Verification items for the finished model (mm, model axes). A direction names the side the tool comes from. Give positions to 0.01 mm unless a question says otherwise; leave off trailing zeros. Loops run counter-clockwise (first coordinate to the right, second up) from the corner with the lowest first, then second, coordinate; pieces in that order, holes last. Notation, with made-up numbers: (43, 40) -> (82, 40) arc R6 cw to (82, 47) -> close; hole circle Ø5 at (19.25, -8). An arc over 180 degrees is marked (long way). Answer in a Markdown table with one row per item. Add a question column.
Q1. Section check A-A on z = 0. Enter the section's corners in (x, y).
Q2. Material ranges on probe 1 along Y at (x, z) = (-9, 0); probe 2 along Y at (x, z) = (9.5, -15.5); probe 3 along X at (y, z) = (4.75, -3), recorded low to high.
Q3. Section check D-D on x = 5. Enter the section's corners in (y, z).
Q4. Gauge pin test, flat ends, axial feed: P1, Ø5, axis at y = 13, z = 0, coming from the +X side; P2, Ø6, axis at x = 10, y = 12.5, coming from the -Z side; P3, Ø5, axis at y = 13, z = 0, coming from the -X side. Record the tip position at first contact, or that the pin passes through.
Q5. Section check B-B on y = 13. Enter the section's corners in (x, z).
Q6. Section check C-C on x = 0. Enter the section's corners in (y, z), and give its area (3 significant figures).
Q7. Release check for a two-part mould opening along Z. For faces 1 (the face through (-5, 0, 0)), 2 (the face through (-7.78, 4.94, 18.75)), 3 (the face through (-3.549, 8.112, 1.846)) record: pulls with the +Z half, pulls with the -Z half, needs draft (parallel to the pull), parting line crosses it, or undercut.
Q8. Set-up check for faces 4 (the face through (-0.325, 11.536, 8.043)), 5 (the face through (9, 10, 9)), 6 (the face through (-18, 9, -10)): record each of +Z, -Z, +X, -X, +Y, -Y from which the full face is reachable in a straight line by a thin tool's end or side.
```python
from build123d import *

# Parameters (mm, degrees)
SKETCH_2_R               = 21.8
EXTRUDE_1_DEPTH          = 16
SKETCH_3_R               = 4
CUT_EXTRUDE_1_DEPTH      = 35.734420968
SKETCH_4_OUTSIDE_W       = 58.34
SKETCH_4_OUTSIDE_H       = 58.34
SKETCH_4_OUTSIDE_R       = 12.5
CUT_EXTRUDE_2_DEPTH      = 6
SKETCH_5_OUTSIDE_W       = 58.34
SKETCH_5_OUTSIDE_H       = 58.34
SKETCH_5_OUTSIDE_R       = 20.3
CUT_EXTRUDE_3_DEPTH      = 8
CUT_EXTRUDE_4_DEPTH      = 35.734420968
CUT_EXTRUDE_4_DEPTH_BACK = 35.734420968
SKETCH_6_R               = 1.5
CUT_EXTRUDE_5_DEPTH      = 35.734421014
CUT_EXTRUDE_5_DEPTH_BACK = 35.734421014
SKETCH_7_R               = 1.5


with BuildPart() as part:
    # 草图2 → 凸台-拉伸1 (new body)
    with BuildSketch(Plane(origin=(0, 0, 0), x_dir=(1, 0, 0), z_dir=(0, 1, 0))):
        with Locations(Location((0, 0, 0), (0, 0, 270))):
            Circle(SKETCH_2_R)
    extrude(amount=EXTRUDE_1_DEPTH)

    # 草图3 → 切除-拉伸1 (cut, through all)
    with BuildSketch(Plane(origin=(0, 16, 0), x_dir=(1, 0, 0), z_dir=(0, 1, 0))):
        with Locations(Location((0, 0, 0), (0, 0, 270))):
            Circle(SKETCH_3_R)
    extrude(amount=-CUT_EXTRUDE_1_DEPTH, mode=Mode.SUBTRACT)

    # 草图4 outside → 切除-拉伸2 (cut)
    with BuildSketch(Plane(origin=(0, 16, 0), x_dir=(1, 0, 0), z_dir=(0, 1, 0))):
        Rectangle(SKETCH_4_OUTSIDE_W, SKETCH_4_OUTSIDE_H)
        with Locations(Location((0, 0, 0), (0, 0, 270))):
            Circle(SKETCH_4_OUTSIDE_R, mode=Mode.SUBTRACT)
    extrude(amount=-CUT_EXTRUDE_2_DEPTH, mode=Mode.SUBTRACT)

    # 草图5 outside → 切除-拉伸3 (cut)
    with BuildSketch(Plane(origin=(0, 1, 0), x_dir=(1, 0, 0), z_dir=(0, 1, 0))):
        Rectangle(SKETCH_5_OUTSIDE_W, SKETCH_5_OUTSIDE_H)
        with Locations(Location((0, 0, 0), (0, 0, 270))):
            Circle(SKETCH_5_OUTSIDE_R, mode=Mode.SUBTRACT)
    extrude(amount=CUT_EXTRUDE_3_DEPTH, mode=Mode.SUBTRACT)

    # 草图6 → 切除-拉伸4 (cut, two sides: drawn at the far end of the back side and taken through both)
    with BuildSketch(Plane(origin=(0, 0, 0), x_dir=(0, 0, -1), z_dir=(1, 0, 0)).offset(-CUT_EXTRUDE_4_DEPTH_BACK)):
        with Locations((0, 13)):
            Circle(SKETCH_6_R)
    extrude(amount=CUT_EXTRUDE_4_DEPTH + CUT_EXTRUDE_4_DEPTH_BACK, mode=Mode.SUBTRACT)

    # 草图7 → 切除-拉伸5 (cut, two sides: drawn at the far end of the back side and taken through both)
    with BuildSketch(Plane.XY.offset(-CUT_EXTRUDE_5_DEPTH_BACK)):
        with Locations((0, 13)):
            Circle(SKETCH_7_R)
    extrude(amount=CUT_EXTRUDE_5_DEPTH + CUT_EXTRUDE_5_DEPTH_BACK, mode=Mode.SUBTRACT)


solid = part.part
```
Taken from the geometry:
| question | item | result |
|---|---|---|
| 1 | outline | (-21.8, 0) -> (-4, 0) -> (-4, 11.5) -> (-12.5, 11.5) -> (-12.5, 10) -> (-21.8, 10) -> (-21.8, 9) -> (-20.3, 9) -> (-20.3, 1) -> (-21.8, 1) -> close; (-12.5, 14.5) -> (-4, 14.5) -> (-4, 16) -> (-12.5, 16) -> close; (4, 0) -> (21.8, 0) -> (21.8, 1) -> (20.3, 1) -> (20.3, 9) -> (21.8, 9) -> (21.8, 10) -> (12.5, 10) -> (12.5, 11.5) -> (4, 11.5) -> close; (4, 14.5) -> (12.5, 14.5) -> (12.5, 16) -> (4, 16) -> close |
| 2 | probe 1 | y = 0 to 11.5, 14.5 to 16 |
| 2 | probe 2 | y = 0 to 10 |
| 2 | probe 3 | x = -20.08 to -2.65, 2.65 to 20.08 |
| 3 | outline | (0, -21.22) -> (1, -21.22) -> (1, -19.67) -> (9, -19.67) -> (9, -21.22) -> (10, -21.22) -> (10, -11.46) -> (16, -11.46) -> (16, 11.46) -> (10, 11.46) -> (10, 21.22) -> (9, 21.22) -> (9, 19.67) -> (1, 19.67) -> (1, 21.22) -> (0, 21.22) -> close; hole circle Ø3 at (13, 0) |
| 4 | P1 | stops at x = 12.5 |
| 4 | P2 | stops at z = -20.14 |
| 4 | P3 | stops at x = -12.5 |
| 5 | outline | (-12.41, -1.5) arc R12.5 ccw to (-1.5, -12.41) -> (-1.5, -3.71) arc R4 cw to (-3.71, -1.5) -> close; (-12.41, 1.5) -> (-3.71, 1.5) arc R4 cw to (-1.5, 3.71) -> (-1.5, 12.41) arc R12.5 ccw to start; (1.5, -12.41) arc R12.5 ccw to (12.41, -1.5) -> (3.71, -1.5) arc R4 cw to (1.5, -3.71) -> close; (1.5, 3.71) arc R4 cw to (3.71, 1.5) -> (12.41, 1.5) arc R12.5 ccw to (1.5, 12.41) -> close |
| 6 | outline | (0, -21.8) -> (1, -21.8) -> (1, -20.3) -> (9, -20.3) -> (9, -21.8) -> (10, -21.8) -> (10, -12.5) -> (11.5, -12.5) -> (11.5, -4) -> (0, -4) -> close; (0, 4) -> (11.5, 4) -> (11.5, 12.5) -> (10, 12.5) -> (10, 21.8) -> (9, 21.8) -> (9, 20.3) -> (1, 20.3) -> (1, 21.8) -> (0, 21.8) -> close; (14.5, -12.5) -> (16, -12.5) -> (16, -4) -> (14.5, -4) -> close; (14.5, 4) -> (16, 4) -> (16, 12.5) -> (14.5, 12.5) -> close |
| 6 | area | 383 mm² |
| 7 | face 1 | needs draft |
| 7 | face 2 | parting line crosses it |
| 7 | face 3 | undercut |
| 8 | face 4 | +Z, -Z |
| 8 | face 5 | +Y |
| 8 | face 6 | none |
